Read the model definition and answer for the solid it produces. Units are mm, in the model's axes. Coordinates: 2 decimals unless noted, no trailing zeros. Write each loop counter-clockwise with the first axis right and the second up, starting at its lowest first coordinate (ties: lowest second). Pieces come first, ordered by that corner, then holes. Notation, with made-up numbers: (82, 7) -> (121, 7) arc R33 ccw to (121, 45) -> close; hole circle Ø1 at (72, 52.25). An arc over 180 degrees is marked (long way). Write item = value, one per line. Start each with the question number.
1) Section D-D (z = 1167.5) is taken. Determine the outline of the cut face in (x, y).
2) Section A-A (z = 991.5) is taken. Determine the outline of the cut face in (x, y).
3) Section B-B (x = 13.25) is taken. Determine the outline of the cut face in (y, z), plus the area to 3 significant figures.
4) Section C-C (y = -360) is taken. Determine the outline of the cut face in (x, z).
5) For a pull along Y with two mould halves and no side action, classify faces 1 (the face through (9.86, -809.151, 752.144)), 2 (the face through (9.86, -906.8, 523.54)), 3 (the face through (9.86, -1563.7, 937.21)) as released by +Y, released by -Y, zero draft, split by the parting line, or undercut.
6) Find the intervals of material crossed by line 1 along Y through (x, z) = (4, 161); line 2 along Y through (x, z) = (3.25, 900); line 3 along Z through (x, y) = (14.5, -1454.5), in increasing order. Write a range as from..to.
7) Flat-ended cylindrical pins translate along their axes: pin 1 Ø12 at (x, z) = (16, 713) entering from -Y; pin 2 Ø5 at (x, z) = (13, 1090) entering from +Y; pin 3 Ø10 at (x, y) = (18, -1269.5) entering from +Z. Find the tip coordinate at first contact, or state that the pin passes through.
from build123d import *

# Parameters (mm, degrees)
BOSS_EXTRUDE1_DEPTH = 20
SKETCH2_R           = 50
CUT_EXTRUDE4_DEPTH  = 2239.523130199
SKETCH3_R           = 50
CUT_EXTRUDE6_DEPTH  = 2239.523130199


with BuildPart() as part:
    # Sketch1 → Boss-Extrude1 (new body)
    with BuildSketch(Plane(origin=(0, 0, 0), x_dir=(0, 0, -1), z_dir=(1, 0, 0))):
        Polygon((0, 0), (-1061.95, -1839.351355098), (-1275.685069654, -1715.951355098), (-213.735069654, 123.4), align=None)
    extrude(amount=BOSS_EXTRUDE1_DEPTH)

    # Sketch2 → Cut-Extrude4 (cut, through all)
    with BuildSketch(Plane.ZY):
        with Locations((976.888502518, -1533.278698946)):
            Circle(SKETCH2_R)
    extrude(amount=-CUT_EXTRUDE4_DEPTH, mode=Mode.SUBTRACT)

    # Sketch3 → Cut-Extrude6 (cut, through all)
    with BuildSketch(Plane(origin=(20, 0, 0), x_dir=(0, 0, -1), z_dir=(1, 0, 0))):
        with Locations((-132.380349241, -85.096529142)):
            Circle(SKETCH3_R)
    extrude(amount=-CUT_EXTRUDE6_DEPTH, mode=Mode.SUBTRACT)


solid = part.part
Answer key:
q1.outline = (0, -1778.41) -> (20, -1778.41) -> (20, -1528.57) -> (0, -1528.57) -> close
q2.outline = (0, -1717.33) -> (20, -1717.33) -> (20, -1581.1) -> (0, -1581.1) -> close; (0, -1485.46) -> (20, -1485.46) -> (20, -1223.73) -> (0, -1223.73) -> close
q3.outline = (-1839.35, 1061.95) -> (0, 0) -> (123.4, 213.74) -> (-1715.95, 1275.69) -> close; hole circle Ø100 at (-1533.28, 976.89); hole circle Ø100 at (-85.1, 132.38)
q3.area = 508,000 mm^2
q4.outline = (0, 207.85) -> (20, 207.85) -> (20, 492.83) -> (0, 492.83) -> close
q5.face_1 = released by +Y
q5.face_2 = released by -Y
q5.face_3 = undercut
q6.line_1 = -278.86..-126.1, -44.1..92.95
q6.line_2 = -1558.85..-1065.25
q6.line_3 = 839.76..1124.74
q7.pin_1 = -1245.34
q7.pin_2 = -1390.01
q7.pin_3 = 1020.81
